```python
from build123d import *

# Parameters (mm, degrees)
SKETCH1_W           = 15
SKETCH1_H           = 16.25
BOSS_EXTRUDE1_DEPTH = 10
SKETCH2_W           = 11.171160898
SKETCH2_H           = 3.40778749
SKETCH2_H_2         = 3.38965483
CUT_EXTRUDE1_DEPTH  = 10
SKETCH3_W           = 23.87
SKETCH3_H           = 18.64
BOSS_EXTRUDE2_DEPTH = 34
SKETCH4_W           = 18.64
SKETCH4_H           = 21.002535876
BOSS_EXTRUDE3_DEPTH = 3
SKETCH5_R           = 2.94201074
BOSS_EXTRUDE4_DEPTH = 7.65
SKETCH6_R           = 1.5
CUT_EXTRUDE2_DEPTH  = 49.595866638


with BuildPart() as part:
    # Sketch1 → Boss-Extrude1 (new body)
    with BuildSketch(Plane(origin=(0, 0, 0), x_dir=(1, 0, 0), z_dir=(0, 1, 0))):
        Rectangle(SKETCH1_W, SKETCH1_H)
    extrude(amount=-BOSS_EXTRUDE1_DEPTH)

    # Sketch2 → Cut-Extrude1 (cut)
    with BuildSketch(Plane(origin=(0, 0, 0), x_dir=(1, 0, 0), z_dir=(0, 1, 0))):
        with Locations((0, 5.398551248)):
            Rectangle(SKETCH2_W, SKETCH2_H)
        with Locations((0, -3.591791831)):
            Rectangle(SKETCH2_W, SKETCH2_H_2)
    extrude(amount=-CUT_EXTRUDE1_DEPTH, mode=Mode.SUBTRACT)

    # Sketch3 → Boss-Extrude2 (add)
    with BuildSketch(Plane(origin=(0, 0, 0), x_dir=(1, 0, 0), z_dir=(0, 1, 0))):
        Rectangle(SKETCH3_W, SKETCH3_H)
    extrude(amount=BOSS_EXTRUDE2_DEPTH)

    # Sketch4 → Boss-Extrude3 (add)
    with BuildSketch(Plane.ZY.offset(11.935)):
        Rectangle(SKETCH4_W, SKETCH4_H)
    boss_extrude3 = extrude(amount=BOSS_EXTRUDE3_DEPTH)

    # Sketch5 → Boss-Extrude4 (add)
    with BuildSketch(Plane(origin=(0, -10.501267938, 0), x_dir=(-1, 0, 0), z_dir=(0, -1, 0))):
        with Locations((15.461680584, 0)):
            Circle(SKETCH5_R)
    boss_extrude4 = extrude(amount=-BOSS_EXTRUDE4_DEPTH)

    # Mirror1: Boss-Extrude3, Boss-Extrude4 across plane
    add(boss_extrude3.mirror(Plane(origin=(0, 0, 0), x_dir=(0, 0, 1), z_dir=(1, 0, 0))))
    add(boss_extrude4.mirror(Plane(origin=(0, 0, 0), x_dir=(0, 0, 1), z_dir=(1, 0, 0))))

    # Sketch6 → Cut-Extrude2 (cut, symmetric)
    with BuildSketch(Plane(origin=(0, -10, 0), x_dir=(-1, 0, 0), z_dir=(0, -1, 0))):
        with Locations(Location((15.29, 0, 0), (0, 0, 90))):
            Circle(SKETCH6_R)
    cut_extrude2 = extrude(amount=CUT_EXTRUDE2_DEPTH, both=True, mode=Mode.SUBTRACT)

    # Mirror2: Cut-Extrude2 across plane
    add(cut_extrude2.mirror(Plane(origin=(0, 0, 0), x_dir=(0, 0, 1), z_dir=(1, 0, 0))), mode=Mode.SUBTRACT)


solid = part.part
```
Here's how the part is built. I have some questions about the finished solid (model axes, mm). A direction names the side the tool comes from. Round coordinates to 2 decimals unless told otherwise and drop trailing zeros. Order: outer loops, then holes, each group sorted by start corner. A loop starts at its lowest first (then second) coordinate and runs counter-clockwise, first axis right, second up. Notation, with made-up numbers: M 53.5,48.25 L 68.5,48.25 A7 ccw 68.5,54.25 Z; hole C 19.5,60.5 d9. An arc over 180 degrees is marked long. Answer in a Markdown table with one row per item.
Item 1: Imagine slicing it at A-A, the plane y = -1. Write out the boundary of the cut face in (x, z) (3 decimals).
A:
| item | result |
|---|---|
| outline | M -14.935,-9.32 L -11.935,-9.32 L -11.935,9.32 L -14.935,9.32 L -14.935,1.457 A1.5 cw -14.935,-1.457 Z; M -7.5,-8.125 L 7.5,-8.125 L 7.5,8.125 L -7.5,8.125 Z; M 11.935,-9.32 L 14.935,-9.32 L 14.935,-1.457 A1.5 cw 14.935,1.457 L 14.935,9.32 L 11.935,9.32 Z; hole M -5.586,-7.102 L 5.586,-7.102 L 5.586,-3.695 L -5.586,-3.695 Z; hole M -5.586,1.897 L 5.586,1.897 L 5.586,5.287 L -5.586,5.287 Z |
Item 2: Imagine slicing it at C-C, the plane x = 5. Write out the boundary of the cut face in (y, z) (3 decimals).
A:
| item | result |
|---|---|
| outline | M -10,-8.125 L 0,-8.125 L 0,-9.32 L 34,-9.32 L 34,9.32 L 0,9.32 L 0,8.125 L -10,8.125 L -10,5.287 L 0,5.287 L 0,1.897 L -10,1.897 L -10,-3.695 L 0,-3.695 L 0,-7.102 L -10,-7.102 Z |
Item 3: Thinking about a two-plate mould opening in Z: for faces 4 (the face through (-13, 10.501, 0)), 5 (the face through (0, -5, -8.125)), 6 (the face through (-5.586, -5, -5)), which applies, +Z half, -Z half, draft (parallel to the pull), parting line (faces both ways), or undercut?
A:
| item | result |
|---|---|
| face 4 | draft |
| face 5 | -Z half |
| face 6 | undercut |
Item 4: If I drill on L1, parallel to X at y = -5, z = 5.5 (3 decimals); L2, parallel to X at y = -2.5, z = 0 (3 decimals); L3, parallel to X at y = -5.25, z = 0 (3 decimals), over which ranges is the centre line in solid material (lowest first)? Write a range as from..to.
A:
| item | result |
|---|---|
| L1 | x = -14.935..-11.935, -7.5..7.5, 11.935..14.935 |
| L2 | x = -13.79..-11.935, -7.5..7.5, 11.935..13.79 |
| L3 | x = -18.404..-16.79, -13.79..-11.935, -7.5..7.5, 11.935..13.79, 16.79..18.404 |
Item 5: I'm going to push flat-ended pins straight in: pin 1 (5 mm diameter, centred on y = 29.5, z = -3, fed in from +X) (3 decimals); pin 2 (3.5 mm diameter, centred on x = -14, z = 1.5, fed in from +Y); pin 3 (1 mm diameter, centred on x = 2, z = 4, fed in from -Y); pin 4 (5 mm diameter, centred on x = 13.5, y = 16, fed in from -Z). Where does each tip first touch, or does it pass through?
A:
| item | result |
|---|---|
| pin 1 | stops at x = 11.935 |
| pin 2 | stops at y = 10.5 |
| pin 3 | stops at y = 0 |
| pin 4 | stops at z = -9.32 |
Item 6: Imagine slicing it at B-B, the plane z = 0. Write out the boundary of the cut face in (x, y) (3 decimals), and give its area (3 significant figures).
A:
| item | result |
|---|---|
| outline | M -18.404,-10.501 L -16.79,-10.501 L -16.79,-2.851 L -18.404,-2.851 Z; M -13.79,-10.501 L -11.935,-10.501 L -11.935,0 L -7.5,0 L -7.5,-10 L 7.5,-10 L 7.5,0 L 11.935,0 L 11.935,-10.501 L 13.79,-10.501 L 13.79,10.501 L 11.935,10.501 L 11.935,34 L -11.935,34 L -11.935,10.501 L -13.79,10.501 Z; M 16.79,-10.501 L 18.404,-10.501 L 18.404,-2.851 L 16.79,-2.851 Z |
| area | 1,060 mm2 |
Item 7: For faces 1 (the face through (-11.935, 22, 0)), 2 (the face through (-7.5, -5, 0)), 3 (the face through (13, 10.501, 0)), which set-ups out of +Z, -Z, +X, -X, +Y, -Y let a thin tool reach every point of the face, with its end or its side?
A:
| item | result |
|---|---|
| face 1 | +Z, -Z, -X, +Y |
| face 2 | +Z, -Z, -Y |
| face 3 | +Z, -Z, +X, +Y |
Item 8: Imagine slicing it at D-D, the plane y = -6.5. Write out the boundary of the cut face in (x, z) (3 decimals), and give its area (3 significant figures).
A:
| item | result |
|---|---|
| outline | M -14.935,-9.32 L -11.935,-9.32 L -11.935,9.32 L -14.935,9.32 L -14.935,2.894 A2.942 ccw long -14.935,-2.894 Z; M -7.5,-8.125 L 7.5,-8.125 L 7.5,8.125 L -7.5,8.125 Z; M 11.935,-9.32 L 14.935,-9.32 L 14.935,-2.894 A2.942 ccw long 14.935,2.894 L 14.935,9.32 L 11.935,9.32 Z; hole C -15.29,0 d3; hole M -5.586,-7.102 L 5.586,-7.102 L 5.586,-3.695 L -5.586,-3.695 Z; hole M -5.586,1.897 L 5.586,1.897 L 5.586,5.287 L -5.586,5.287 Z; hole C 15.29,0 d3 |
| area | 299 mm2 |
